Autodesk Inventor part; units mm, degrees
ref_plane "YZ Plane" through (0, 0, 0) normal (1, 0, 0) x (0, 1, 0)
ref_plane "XZ Plane" through (0, 0, 0) normal (0, 1, 0) x (-1, 0, 0)
ref_plane "XY Plane" through (0, 0, 0) normal (0, 0, 1) x (1, 0, 0)
sketch "Sketch1" plane through (0, 0, 0) normal (0, 1, 0) x (-1, 0, 0)
  line L0 (0, 0) -> (-16.25, 0)
  line L1 (0, 0) -> (46.75, 0)
  line L2 (300, 0) -> (330, 0)
  line L3 (330, 30) -> (-30, 30)
  line L4 (-16.25, 15.5) -> (46.75, 15.5)
  line L5 (46.75, 15.5) -> (46.75, 0)
  line L6 (46.75, -15.5) -> (-16.25, -15.5)
  line L7 (-16.25, -15.5) -> (-16.25, 0)
  line L8 (-16.25, 15.5) -> (46.75, -15.5) construction
  line L9 (46.75, 15.5) -> (-16.25, -15.5) construction
  line L10 (-19.25, 8.5) -> (49.75, 8.5) construction
  line L11 (49.75, 8.5) -> (49.75, -8.5) construction
  line L12 (49.75, -8.5) -> (-19.25, -8.5) construction
  line L13 (-19.25, -8.5) -> (-19.25, 8.5) construction
  line L14 (-19.25, 8.5) -> (49.75, -8.5) construction
  line L15 (49.75, 8.5) -> (-19.25, -8.5) construction
  line L16 (-30, 0) -> (-30, 30)
  line L17 (330, 0) -> (330, 30)
  line L18 (46.75, 0) -> (300, 0)
  line L19 (46.75, 0) -> (46.75, -15.5)
  line L20 (-16.25, 0) -> (-30, 0)
  line L21 (-16.25, 0) -> (-16.25, 15.5)
  line L22 (300, 0) -> (300, 18.5) construction
  line L23 (0, 0) -> (-30, 0) construction
  point P0 (15.25, 0)
  point P1 (15.25, 0)
  point P2 (285, 0)
  dimension "d0" = 300
  dimension "d5" = 63
  dimension "d6" = 31
  dimension "d7" = 69
  dimension "d8" = 17
  dimension "d9" = 16.25
  dimension "d10" = 30
  dimension "d11" = 30
  dimension "d20" = 18.5
  dimension "d21" = 15
extrude "Extrusion1" add sketch "Sketch1" along normal blind 6 contours L20 L16 L3 L17 L2 L18 L5 L4 L21
hole "Hole1" at (19.25, 0, 8.5) at (-49.75, 0, 8.5) direction (0, 1, 0) diameter 2 end through all
hole "Hole2" at (-300, 0, 0) at (-300, 0, 18.5) at (-285, 0, 0) direction (0, 1, 0) diameter 3 end through all
fillet "Fillet1" radius 20 1 edges at (30, 3, 30)
mirror "Mirror1" about plane through (-46.75, 0, 0) normal (0, 0, -1)
properties part number "segment1a" material "Plywood, Finish"
Check sheet for the modelled part. Datum: model origin and axes. Units: mm. A direction names the side the tool comes from. Round coordinates to 2 decimals unless told otherwise and drop trailing zeros. Write each loop counter-clockwise with the first axis right and the second up, starting at its lowest first coordinate (ties: lowest second). Pieces come first, ordered by that corner, then holes. Notation, with made-up numbers: M 89,-8.75 L 134,-8.75 A35 ccw 134,30.25 Z; hole C 33.25,-7.5 d3. An arc over 180 degrees is marked long. Write item = value, one per line. Start each with the question number.
1. Release check for a two-part mould opening along Z. For faces 3 (the flat face through (-15, 3, 15.5)), 4 (the cylindrical face through (23.986, 3.042, 24.297)), 5 (the flat face through (16.25, 3, 0)), 6 (the flat face through (30, 3, 0)) record: pulls with the +Z half, pulls with the -Z half, needs draft (parallel to the pull), parting line crosses it, or undercut.
2. Gauge pin test, flat end, axial feed: pin 1 (1.8 mm diameter, centred on x = -49.75, z = 8.5, fed in from +Y). Record the tip position at first contact, or that the pin passes through.
3. Section check B-B, the plane y = 1.4. State how many separate pieces and enclosed holes the cut face has, then the cut area to 3 significant figures.
4. Section check A-A, the plane x = -4. Record the cut outline in (y, z).
5. Tool access check on faces 1 (the cylindrical face through (24.297, 3.042, -23.986)), 2 (the flat face through (-16, 3, -15.5)). Record the directions out of +Z, -Z, +X, -X, +Y, -Y that give a thin tool (end or side, any length) a straight path to the whole face; none if there is none.
6. Scan lines: line 1 (X direction, y = 2.65, z = -8.5); line 2 (Z direction, x = -49.75, y = 4.4); line 3 (Z direction, x = -300, y = 1.85). Record each from-to range of solid material in increasing order. Write a range as [from, to].
Results found:
q1.face_3 = undercut
q1.face_4 = pulls with the +Z half
q1.face_5 = undercut
q1.face_6 = needs draft
q2.pin_1 = through
q3.separate_pieces = 1
q3.enclosed_holes = 9
q3.area = 19,400 mm^2
q4.outline = M 0,-30 L 6,-30 L 6,-15.5 L 0,-15.5 Z; M 0,15.5 L 6,15.5 L 6,30 L 0,30 Z
q5.face_1 = -Z, +X, +Y, -Y
q5.face_2 = +Y, -Y
q6.line_1 = [-330, -50.75], [-48.75, -46.75], [16.25, 18.25], [20.25, 30]
q6.line_2 = [-30, -9.5], [-7.5, 7.5], [9.5, 30]
q6.line_3 = [-30, -20], [-17, -1.5], [1.5, 17], [20, 30]
